```python
from build123d import *

# Parameters (mm, degrees)
SKETCH_1_R               = 12.5
SKETCH_1_R_2             = 6
EXTRUDE_1_DEPTH          = 10
SKETCH_2_R               = 2.5
CUT_EXTRUDE_1_DEPTH      = 10
CUT_EXTRUDE_1_DEPTH_BACK = 13.5


with BuildPart() as part:
    # 草图1 → 凸台-拉伸1 (new body)
    with BuildSketch(Plane.XY):
        Circle(SKETCH_1_R)
        Circle(SKETCH_1_R_2, mode=Mode.SUBTRACT)
    extrude(amount=EXTRUDE_1_DEPTH)

    # 草图2 → 切除-拉伸1 (cut, two sides)
    with BuildSketch(Plane(origin=(0, 0, 0), x_dir=(1, 0, 0), z_dir=(0, 1, 0))) as cut_extrude_1_sk:
        with Locations((0, -5)):
            Circle(SKETCH_2_R)
    extrude(amount=CUT_EXTRUDE_1_DEPTH, mode=Mode.SUBTRACT)
    extrude(cut_extrude_1_sk.sketch, amount=-CUT_EXTRUDE_1_DEPTH_BACK, mode=Mode.SUBTRACT)


solid = part.part
```
Here's how the part is built. I have some questions about the finished solid (model axes, mm). A direction names the side the tool comes from. Round coordinates to 2 decimals unless told otherwise and drop trailing zeros. Order: outer loops, then holes, each group sorted by start corner. A loop starts at its lowest first (then second) coordinate and runs counter-clockwise, first axis right, second up. Notation, with made-up numbers: (29.5, 4.25) -> (66.5, 4.25) arc R28 cw to (66.5, 28.25) -> close; hole circle Ø1 at (-27, 40.5). An arc over 180 degrees is marked (long way). Use a Markdown table: item, result. Add a question column.
(1) For faces 4 (the face through (11.923, 3.755, 4.93)), 5 (the face through (-2.5, -8.9, 4.9)), which set-ups out of +Z, -Z, +X, -X, +Y, -Y let a thin tool reach every point of the face, with its end or its side?
(2) If we mould it in two halves opening along Z, with no side actions, what happens to faces 1 (the face through (-0.54, 7.7, 7.44)), 2 (the face through (-3, -5.4, 10)), 3 (the face through (-3, -5.4, 0))? For each: released by +Z, released by -Z, zero draft, split by the parting line, or undercut.
(3) Suppose I cut it at A-A, the plane x = 0. Please give me the cut outline in (y, z).
(4) Suppose I cut it at D-D, the plane y = -4.5. Please give me the cut outline in (x, z).
(5) For pin 1 Ø2 at (y, z) = (9, 3.5) entering from -X; pin 2 Ø4 at (x, z) = (5, 8) entering from +Y; pin 3 Ø1 at (x, z) = (-8.5, 1.5) entering from -Y, each with a flat end and sliding along its axis, tell me the tip position at first contact or that it passes through.
(6) Suppose I cut it at C-C, the plane z = 1. Please give me the cut outline in (x, y), and give its area (3 significant figures).
(7) I need wall thicknesses on line 1 along Z through (x, y) = (0, -9.25); line 2 along X through (y, z) = (8.5, 6.25); line 3 along Y through (x, z) = (-5.5, 2.5). Which ranges of each line are inside material? Lowest first, please.
(8) Suppose I cut it at B-B, the plane y = 0. Please give me the cut outline in (x, z), and give its area (3 significant figures).
Verdict:
| question | item | result |
|---|---|---|
| 1 | face 4 | +Z, -Z |
| 1 | face 5 | -Y |
| 2 | face 1 | undercut |
| 2 | face 2 | released by +Z |
| 2 | face 3 | released by -Z |
| 3 | outline | (-12.5, 0) -> (-6, 0) -> (-6, 2.5) -> (-12.5, 2.5) -> close; (-12.5, 7.5) -> (-6, 7.5) -> (-6, 10) -> (-12.5, 10) -> close; (6, 0) -> (12.5, 0) -> (12.5, 10) -> (6, 10) -> (6, 7.5) -> (10, 7.5) -> (10, 2.5) -> (6, 2.5) -> close |
| 4 | outline | (-11.66, 0) -> (-3.97, 0) -> (-3.97, 10) -> (-11.66, 10) -> close; (3.97, 0) -> (11.66, 0) -> (11.66, 10) -> (3.97, 10) -> close |
| 5 | pin 1 | x = -9.6 |
| 5 | pin 2 | y = 12.13 |
| 5 | pin 3 | y = -9.6 |
| 6 | outline | circle Ø25 at (0, 0); hole circle Ø12 at (0, 0) |
| 6 | area | 378 mm2 |
| 7 | line 1 | 0 to 2.5, 7.5 to 10 |
| 7 | line 2 | -9.17 to -2.17, 2.17 to 9.17 |
| 7 | line 3 | -11.22 to -2.4, 2.4 to 11.22 |
| 8 | outline | (-12.5, 0) -> (-6, 0) -> (-6, 10) -> (-12.5, 10) -> close; (6, 0) -> (12.5, 0) -> (12.5, 10) -> (6, 10) -> close |
| 8 | area | 130 mm2 |
